```python
from build123d import *

# Parameters (mm, degrees)
F0_R     = 9.525
F0_R_2   = 12.7
F1_DEPTH = 25.4
F2_R     = 2.38125
F3_DEPTH = 9.526
F4_R     = 2.38125
F5_DEPTH = 38.101


with BuildPart() as f1:
    # F0 (on Front) → F1 (new body)
    with BuildSketch(Plane.XZ):
        Polygon((-76.2, 0), (0, 0), (0, 9.525), (-38.1, 9.525), (-38.1, 71.4375), (-76.2, 71.4375), align=None)
        with Locations((-57.15, 25.4)):
            Circle(F0_R, mode=Mode.SUBTRACT)
        with Locations((-57.15, 52.3875)):
            Circle(F0_R_2, mode=Mode.SUBTRACT)
    extrude(amount=F1_DEPTH)

    # F2 (on face) → F3 (cut, through all)
    with BuildSketch(Plane.XY.offset(9.525)):
        with Locations((-7.14375, -12.7)):
            Circle(F2_R)
        with Locations((-19.84375, -12.7)):
            Circle(F2_R)
    extrude(amount=-F3_DEPTH, mode=Mode.SUBTRACT)

    # F4 (on face) → F5 (cut, through all)
    with BuildSketch(Plane.YZ.offset(-38.1)):
        with Locations((-12.7, 25.4)):
            Circle(F4_R)
        with Locations((-12.7, 52.3875)):
            Circle(F4_R)
    extrude(amount=-F5_DEPTH, mode=Mode.SUBTRACT)


solid = f1.part
```
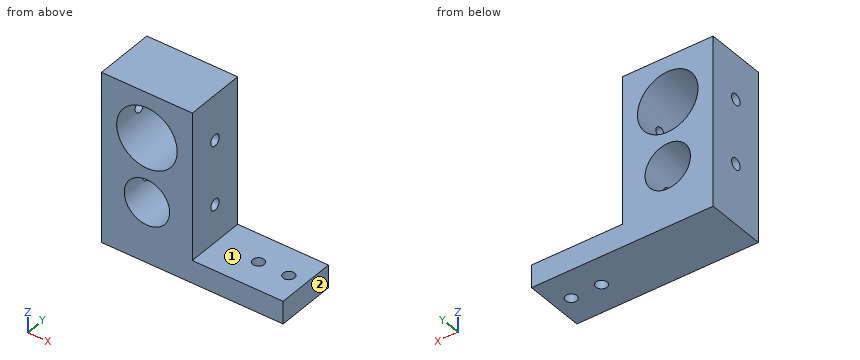
Verification items for the finished model (mm, model axes). Face numbers are marked on the shaded views. A direction names the side the tool comes from. Coordinates: 2 decimals unless noted, no trailing zeros. Loops run counter-clockwise (first coordinate to the right, second up) from the corner with the lowest first, then second, coordinate; pieces in that order, holes last. Notation, with made-up numbers: (89, 47.5) - (99, 47.5) arc R21 cw to (99, 73.5) - close; hole circle Ø5 at (-17.5, 68.25). An arc over 180 degrees is marked (long way). Return JSON: item names as keys, results as strings.
1. Section check C-C, the plane x = -57.15. Record the boundary of the cut face in (y, z) (1 decimal).
Established:
{"outline": "(-25.4, 0) - (0, 0) - (0, 15.9) - (-25.4, 15.9) - close; (-25.4, 34.9) - (0, 34.9) - (0, 39.7) - (-25.4, 39.7) - close; (-25.4, 65.1) - (0, 65.1) - (0, 71.4) - (-25.4, 71.4) - close"}
2. Thickness scan on L1, parallel to Z at x = -73.5, y = -12.7; L2, parallel to Z at x = -57, y = -13.25; L3, parallel to Z at x = -19.5, y = -22.5 (3 decimals). Record the ranges inside material, lowest first.
Established:
{"L1": "z = 0 to 23.02, 27.78 to 50.01, 54.77 to 71.44", "L2": "z = 0 to 15.88, 34.92 to 39.69, 65.09 to 71.44", "L3": "z = 0 to 9.525"}
3. Go/stop test with flat-tipped pins: pin 1 (4 mm diameter, centred on y = -12.7, z = 25.4, fed in from +X); pin 2 (12.5 mm diameter, centred on x = -28.5, y = -11.5, fed in from +Z) (3 decimals); pin 3 (6 mm diameter, centred on y = -5, z = 24, fed in from +X). Record where each tip stops, or that it passes through.
Established:
{"pin 1": "passes through", "pin 2": "stops at z = 9.525", "pin 3": "stops at x = -38.1"}
4. Section check B-B, the plane z = 25.4. Record the boundary of the cut face in (x, y) (3 decimals), then the cut area to 3 significant figures.
Established:
{"outline": "(-76.2, -25.4) - (-66.675, -25.4) - (-66.675, -15.081) - (-76.2, -15.081) - close; (-76.2, -10.319) - (-66.675, -10.319) - (-66.675, 0) - (-76.2, 0) - close; (-47.625, -25.4) - (-38.1, -25.4) - (-38.1, -15.081) - (-47.625, -15.081) - close; (-47.625, -10.319) - (-38.1, -10.319) - (-38.1, 0) - (-47.625, 0) - close", "area": "393 mm2"}
5. Tool access check on the marked faces 1 and 2. Record the directions out of +Z, -Z, +X, -X, +Y, -Y that give a thin tool (end or side, any length) a straight path to the whole face; none if there is none.
Established:
{"face 1": "+Z, +X, +Y, -Y", "face 2": "+Z, -Z, +X, +Y, -Y"}
6. Section check A-A, the plane y = -12.7. Count the separate pieces of the cut face and the enclosed holes in it, then the cut area to 3 significant figures.
Established:
{"separate pieces": "5", "enclosed holes": "0", "area": "2,050 mm2"}
